Geometry check sheet. Reference: the model listing, model coordinates, mm. A direction names the side the tool comes from. Round coordinates to 2 decimals unless told otherwise and drop trailing zeros. Order: outer loops, then holes, each group sorted by start corner. A loop starts at its lowest first (then second) coordinate and runs counter-clockwise, first axis right, second up. Notation, with made-up numbers: M 78.25,-36.5 L 85.25,-36.5 A17 cw 85.25,-18.5 Z; hole C 4.25,57.5 d4. An arc over 180 degrees is marked long. Answer as a JSON object with one key per item and string values. Group by question number.
```python
from build123d import *

# Parameters (mm, degrees)
CROQUIS1_R                   = 2.5
SALIENTE_EXTRUIR1_DEPTH      = 5
SALIENTE_EXTRUIR2_DEPTH      = 5.5
SALIENTE_EXTRUIR5_DEPTH      = 2
SALIENTE_EXTRUIR5_DEPTH_BACK = 0.1
CROQUIS2_W                   = 41.5
CROQUIS2_H                   = 8
CROQUIS2_H_2                 = 4
CROQUIS2_W_2                 = 4
CROQUIS3_R                   = 2
SALIENTE_EXTRUIR6_DEPTH      = 7.5
CORTAR_EXTRUIR1_REACH        = 39.167
CROQUIS3_3_R                 = 2
CORTAR_EXTRUIR2_START        = -3
CROQUIS4_R                   = 3.5
CROQUIS4_R_2                 = 2
CORTAR_EXTRUIR2_DEPTH        = 3
REDONDEO1_R                  = 2
REDONDEO4_R                  = 2
REDONDEO3_R                  = 1


with BuildPart() as part:
    # Croquis1 → Saliente-Extruir1 (new body)
    with BuildSketch(Plane(origin=(0, 0, 0), x_dir=(1, 0, 0), z_dir=(0, 1, 0))):
        with BuildLine():
            Line((-24.75, -24.75), (24.75, -24.75))
            Line((24.75, -24.75), (24.75, -20.75))
            Line((24.75, -20.75), (-4, -20.75))
            ThreePointArc((-4, -20.75), (-7.5, -17.25), (-4, -13.75))
            Line((-4, -13.75), (24.75, -13.75))
            Line((24.75, -13.75), (24.75, 24.75))
            Line((24.75, 24.75), (-24.75, 24.75))
            Line((-24.75, 24.75), (-24.75, 20.75))
            Line((-24.75, 20.75), (4, 20.75))
            ThreePointArc((4, 20.75), (7.5, 17.25), (4, 13.75))
            Line((4, 13.75), (-24.75, 13.75))
            Line((-24.75, 13.75), (-24.75, -24.75))
        make_face()
        with Locations(Location((0, 0, 0), (0, 0, 270))):
            Circle(CROQUIS1_R, mode=Mode.SUBTRACT)
    extrude(amount=-SALIENTE_EXTRUIR1_DEPTH)

    # Croquis1<3> → Saliente-Extruir2 (add)
    with BuildSketch(Plane(origin=(0, 0, 0), x_dir=(1, 0, 0), z_dir=(0, 1, 0))):
        Polygon((-24.75, 8.75), (-24.75, -24.75), (24.75, -24.75), (24.75, -20.75), (-4, -20.75), (-20.75, -20.75), (-20.75, 8.75), align=None)
        Polygon((-24.75, 24.75), (-24.75, 20.75), (4, 20.75), (20.75, 20.75), (20.75, -8.75), (24.75, -8.75), (24.75, 24.75), align=None)
    extrude(amount=SALIENTE_EXTRUIR2_DEPTH)

    # Croquis2 → Saliente-Extruir5 (add, two sides: drawn at the far end of the back side and taken through both)
    with BuildSketch(Plane(origin=(0, 5.5, 0), x_dir=(1, 0, 0), z_dir=(0, 1, 0)).offset(-SALIENTE_EXTRUIR5_DEPTH_BACK)):
        with Locations((0, 20.75)):
            Rectangle(CROQUIS2_W, CROQUIS2_H)
        Polygon((-20.75, 24.75), (-24.75, 24.75), (-24.75, 8.75), (-20.75, 8.75), (-20.75, 16.75), align=None)
        with Locations((0, -18.75)):
            Rectangle(CROQUIS2_W, CROQUIS2_H_2)
        with Locations((0, -22.75)):
            Rectangle(CROQUIS2_W, CROQUIS2_H_2)
        Polygon((-20.75, 8.75), (-24.75, 8.75), (-24.75, -24.75), (-20.75, -24.75), (-20.75, -20.75), (-20.75, -16.75), align=None)
        Polygon((24.75, 24.75), (20.75, 24.75), (20.75, 16.75), (20.75, -16.75), (20.75, -20.75), (24.75, -20.75), align=None)
        with Locations((22.75, -22.75)):
            Rectangle(CROQUIS2_W_2, CROQUIS2_H_2)
    extrude(amount=SALIENTE_EXTRUIR5_DEPTH + SALIENTE_EXTRUIR5_DEPTH_BACK)

    # Croquis3 → Saliente-Extruir6 (add)
    with BuildSketch(Plane(origin=(0, 7.5, 0), x_dir=(1, 0, 0), z_dir=(0, 1, 0))):
        with BuildLine():
            Line((-20.75, 4), (-20.75, -4))
            Line((-20.75, -4), (-17.5, -4))
            ThreePointArc((-17.5, -4), (-13.5, 0), (-17.5, 4))
            Line((-17.5, 4), (-20.75, 4))
        make_face()
        with Locations(Location((-17.5, 0, 0), (0, 0, 270))):
            Circle(CROQUIS3_R, mode=Mode.SUBTRACT)
    saliente_extruir6 = extrude(amount=-SALIENTE_EXTRUIR6_DEPTH)

    # Croquis3<3> → Cortar-Extruir1 (cut, up to next)
    with BuildSketch(Plane(origin=(0, 7.5, 0), x_dir=(1, 0, 0), z_dir=(0, 1, 0)), mode=Mode.PRIVATE) as cortar_extruir1_sk1:
        with Locations(Location((-17.5, 0, 0), (0, 0, 270))):
            Circle(CROQUIS3_3_R)
    cortar_extruir1_tool1 = extrude(cortar_extruir1_sk1.sketch, amount=-CORTAR_EXTRUIR1_REACH, mode=Mode.PRIVATE) & part.part
    cortar_extruir1 = cortar_extruir1_tool1.solids().sort_by_distance((-17.5, 7.5, 0))[0]
    add(cortar_extruir1, mode=Mode.SUBTRACT)

    # Simetría1: Saliente-Extruir6, Cortar-Extruir1 across plane
    add(saliente_extruir6.mirror(Plane(origin=(0, 0, 0), x_dir=(0, 0, 1), z_dir=(1, 0, 0))))
    add(cortar_extruir1.mirror(Plane(origin=(0, 0, 0), x_dir=(0, 0, 1), z_dir=(1, 0, 0))), mode=Mode.SUBTRACT)

    # Croquis4 → Cortar-Extruir2 (cut)
    # profile 1 of 2: a face of its own
    with BuildSketch(Plane.XZ.offset(5).offset(CORTAR_EXTRUIR2_START)):
        with Locations(Location((-17.5, 0, 0), (0, 0, 270))):
            Circle(CROQUIS4_R)
        with Locations(Location((-17.5, 0, 0), (0, 0, 90))):
            Circle(CROQUIS4_R_2, mode=Mode.SUBTRACT)
    # profile 2 of 2: a face of its own
    with BuildSketch(Plane.XZ.offset(5).offset(CORTAR_EXTRUIR2_START)):
        with Locations(Location((17.5, 0, 0), (0, 0, 270))):
            Circle(CROQUIS4_R)
        with Locations(Location((17.5, 0, 0), (0, 0, 90))):
            Circle(CROQUIS4_R_2, mode=Mode.SUBTRACT)
    extrude(amount=CORTAR_EXTRUIR2_DEPTH, mode=Mode.SUBTRACT)

    # Redondeo1
    redondeo1_edges = [part.edges().sort_by_distance(p)[0] for p in [
        (20.75, 6.45, 16.75),
        (-20.75, 6.45, 16.75),
        (20.75, 6.45, -16.75),
        (-20.75, 3.75, -4),
        (-20.75, 3.75, 4),
        (20.75, 3.75, 4),
        (20.75, 3.75, -4),
        (-20.75, 6.45, -16.75),
    ]]
    fillet(redondeo1_edges, radius=REDONDEO1_R)

    # Redondeo4
    redondeo4_edges = [part.edges().sort_by_distance(p)[0] for p in [
        (0, -5, -24.75),
        (-24.75, -5, -22.75),
        (24.75, 1.25, 24.75),
        (-24.75, 1.25, 24.75),
        (-24.75, 1.25, -24.75),
        (24.75, 1.25, -24.75),
        (-24.75, -5, 5.5),
        (0, -5, 24.75),
        (24.75, -5, 22.75),
        (24.75, -5, -5.5),
        (20.75, 2.7, -20.75),
        (-20.75, 2.7, 20.75),
    ]]
    fillet(redondeo4_edges, radius=REDONDEO4_R)

    # Redondeo3
    redondeo3_edges = [part.edges().sort_by_distance(p)[0] for p in [
        (7.5, -5, -17.25),
        (24.75, 1.2, 20.75),
        (24.75, -1.5, 13.75),
        (9.375, -5, 13.75),
        (9.375, -5, 20.75),
        (-9.375, -5, -13.75),
        (-9.375, -5, -20.75),
        (24.164213562, -4.414213562, 13.75),
        (24.164213562, -4.414213562, 20.75),
        (-24.75, -1.5, -13.75),
        (-24.164213562, -4.414213562, -13.75),
        (-24.75, 1.2, -20.75),
        (-24.164213562, -4.414213562, -20.75),
        (-7.5, -5, 17.25),
        (24.75, 2.7, 8.75),
        (20.75, 2.7, 8.75),
        (-24.75, 2.7, -8.75),
        (-20.75, 2.7, -8.75),
    ]]
    fillet(redondeo3_edges, radius=REDONDEO3_R)


solid = part.part
```
1) Go/stop test with flat-tipped pins: P1, Ø4.5, axis at x = 17.5, z = 0, coming from the -Y side; P2, Ø1, axis at x = 8, z = -12.5, coming from the +Y side. Record where each tip stops, or that it passes through.
2) Sectioned sample at A-A (x = 0). Record the boundary of the cut face in (y, z).
3) Sectioned sample at C-C (x = 12.5). Record the boundary of the cut face in (y, z).
4) Sectioned sample at D-D (y = -1). Record the boundary of the cut face in (x, z), then the cut area to 3 significant figures.
5) Sectioned sample at B-B (z = 0). Count the separate pieces of the cut face and the enclosed holes in it, then the cut area to 3 significant figures.
6) Set-up check for faces 1 (the flat face through (-18, 4, 4)), 2 (the cylindrical face through (-20.18, 2.74, 20.15)), 3 (the flat face through (16, -2, -2)), 4 (the flat face through (-23, 3, -8.75)): record each of +Z, -Z, +X, -X, +Y, -Y from which the full face is reachable in a straight line by a thin tool's end or side.
7) Release check for a two-part mould opening along Z. For faces 5 (the cylindrical face through (24.15, 2.32, -24.18)), 6 (the flat face through (-10, -2, -13.75)), 7 (the cylindrical face through (-24.15, -4.43, -22.24)), 8 (the cylindrical face through (-13.5, 3.8, 0.1)) record: +Z half, -Z half, draft (parallel to the pull), parting line (faces both ways), or undercut.
8) Thickness scan on line 1 along X through (y, z) = (0.25, 0); line 2 along X through (y, z) = (-3.75, 0); line 3 along Z through (x, y) = (-7, 5.25). Record the ranges inside material, lowest first. Write a range as [from, to].
Final values:
{
 "1": {"P1": "stops at y = -2", "P2": "stops at y = 0"},
 "2": {"outline": "M -5,-22.75 A2 ccw -3,-24.75 L 7.5,-24.75 L 7.5,-16.75 L 5.4,-16.75 L 5.4,-20.75 L -4,-20.75 A1 ccw -5,-21.75 Z; M -5,-12.75 A1 ccw -4,-13.75 L 0,-13.75 L 0,-2.5 L -5,-2.5 Z; M -5,2.5 L 0,2.5 L 0,13.75 L -4,13.75 A1 ccw -5,12.75 Z; M -5,21.75 A1 ccw -4,20.75 L 5.4,20.75 L 5.4,16.75 L 7.5,16.75 L 7.5,24.75 L -3,24.75 A2 ccw -5,22.75 Z"},
 "3": {"outline": "M -5,-22.75 A2 ccw -3,-24.75 L 7.5,-24.75 L 7.5,-16.75 L 5.4,-16.75 L 5.4,-20.75 L 0,-20.75 L 0,13.75 L -4,13.75 A1 ccw -5,12.75 Z; M -5,21.75 A1 ccw -4,20.75 L 5.4,20.75 L 5.4,16.75 L 7.5,16.75 L 7.5,24.75 L -3,24.75 A2 ccw -5,22.75 Z"},
 "4": {"outline": "M -24.75,-22.75 A2 ccw -22.75,-24.75 L 22.75,-24.75 A2 ccw 24.75,-22.75 L 24.75,12.75 A1 ccw 23.75,13.75 L -4,13.75 A3.5 cw -4,20.75 L 23.75,20.75 A1 ccw 24.75,21.75 L 24.75,22.75 A2 ccw 22.75,24.75 L -22.75,24.75 A2 ccw -24.75,22.75 L -24.75,-12.75 A1 ccw -23.75,-13.75 L 4,-13.75 A3.5 cw 4,-20.75 L -23.75,-20.75 A1 ccw -24.75,-21.75 Z; hole C -17.5,0 d4; hole C 0,0 d5; hole C 17.5,0 d4", "area": "1,960 mm^2"},
 "5": {"separate pieces": "4", "enclosed holes": "0", "area": "272 mm^2"},
 "6": {"face 1": "+Y", "face 2": "+X", "face 3": "-Y", "face 4": "-X"},
 "7": {"face 5": "-Z half", "face 6": "undercut", "face 7": "draft", "face 8": "undercut"},
 "8": {"line 1": "x = [-24.75, -19.5], [-15.5, -13.5], [13.5, 15.5], [19.5, 24.75]", "line 2": "x = [-24.6, -21], [-14, -2.5], [2.5, 14], [21, 24.6]", "line 3": "z = [-24.75, -20.75], [20.75, 24.75]"}
}
